CAD build for the part. Positions are in the model's coordinates, mm. A direction names the side the tool comes from. Round coordinates to 2 decimals unless told otherwise and drop trailing zeros. Order: outer loops, then holes, each group sorted by start corner. A loop starts at its lowest first (then second) coordinate and runs counter-clockwise, first axis right, second up.
```python
from build123d import *

# Parameters (mm, degrees)
SKETCH1_R                = 6.35
BOSS_EXTRUDE1_DEPTH      = 55
BOSS_EXTRUDE1_DEPTH_BACK = 40
SKETCH2_OUTSIDE_W        = 34.036
SKETCH2_OUTSIDE_H        = 34.036
SKETCH2_OUTSIDE_R        = 4.7625
CUT_EXTRUDE1_DEPTH       = 20
SKETCH3_OUTSIDE_W        = 34.036
SKETCH3_OUTSIDE_H        = 34.036
SKETCH3_OUTSIDE_R        = 4.7625
CUT_EXTRUDE2_DEPTH       = 20


with BuildPart() as part:
    # Sketch1 → Boss-Extrude1 (new body, two sides)
    with BuildSketch(Plane(origin=(0, 0, 0), x_dir=(0, 0, -1), z_dir=(1, 0, 0))) as boss_extrude1_sk:
        Circle(SKETCH1_R)
    extrude(amount=BOSS_EXTRUDE1_DEPTH)
    extrude(boss_extrude1_sk.sketch, amount=-BOSS_EXTRUDE1_DEPTH_BACK)

    # Sketch2 outside → Cut-Extrude1 (cut)
    with BuildSketch(Plane.ZY.offset(40)):
        Rectangle(SKETCH2_OUTSIDE_W, SKETCH2_OUTSIDE_H)
        Circle(SKETCH2_OUTSIDE_R, mode=Mode.SUBTRACT)
    extrude(amount=-CUT_EXTRUDE1_DEPTH, mode=Mode.SUBTRACT)

    # Sketch3 outside → Cut-Extrude2 (cut)
    with BuildSketch(Plane(origin=(55, 0, 0), x_dir=(0, 0, -1), z_dir=(1, 0, 0))):
        Rectangle(SKETCH3_OUTSIDE_W, SKETCH3_OUTSIDE_H)
        Circle(SKETCH3_OUTSIDE_R, mode=Mode.SUBTRACT)
    extrude(amount=-CUT_EXTRUDE2_DEPTH, mode=Mode.SUBTRACT)


solid = part.part
```
1. Pin check, flat tips, straight feed: P1, Ø1.5, axis at x = -9.5, z = 4.5, coming from the -Y side; P2, Ø5, axis at x = 22, z = 3.5, coming from the +Y side; P3, Ø3, axis at x = 27.5, y = 2.5, coming from the -Z side. Stop position of each tip, or through.
2. Cut at D-D, the plane x = 0.5. Write the cut outline in (y, z).
3. Drill centre lines: line 1 (X direction, y = -4.75, z = 0.75); line 2 (Z direction, x = 32, y = 0.25); line 3 (Z direction, x = 46, y = -0.5). Where is each one in solid material? Low to high.
4. Cut at A-A, the plane z = 0. Write the cut outline in (x, y).
5. Tool access for faces 1 (the face through (-30.14, -2.9, -3.78)), 2 (the face through (35, 5, -1)), 3 (the face through (7.89, -6.2, 1.38)): list every direction of +Z, -Z, +X, -X, +Y, -Y with a clear straight run to the whole face (end or side of a thin tool).
6. Cut at C-C, the plane x = -32. Write the cut outline in (y, z) (1 decimal), and give its area (3 significant figures).
Outcome:
1. P1: stops at y = -5.12
1. P2: stops at y = 6.27
1. P3: stops at z = -6.27
2. outline: circle Ø12.7 at (0, 0)
3. line 1: x = -20 to 35
3. line 2: z = -6.35 to 6.35
3. line 3: z = -4.74 to 4.74
4. outline: (-40, -4.76) - (-20, -4.76) - (-20, -6.35) - (35, -6.35) - (35, -4.76) - (55, -4.76) - (55, 4.76) - (35, 4.76) - (35, 6.35) - (-20, 6.35) - (-20, 4.76) - (-40, 4.76) - close
5. face 1: -X
5. face 2: +X
5. face 3: +X, -X
6. outline: circle Ø9.5 at (0, 0)
6. area: 71.3 mm2
